Could you check a few things on this model? Use its own coordinates, in mm. Give positions to 0.01 mm unless a question says otherwise; leave off trailing zeros. Order: outer loops, then holes, each group sorted by start corner. A loop starts at its lowest first (then second) coordinate and runs counter-clockwise, first axis right, second up. Notation, with made-up numbers: (58.25, -31) -> (62.25, -31) arc R18 ccw to (62.25, -12) -> close; hole circle Ø11 at (53, -33). An arc over 180 degrees is marked (long way). Answer as CSV lines item,"result". Start each with the question number.
(1) I want a section at A-A (x = 0). Please give me the cut outline in (y, z).
(2) I want a section at B-B (z = 8.5). Please give me the cut outline in (x, y), plus the area to 3 significant figures.
(3) I need wall thicknesses on L1, parallel to Z at x = 0, y = -2.25; L2, parallel to X at y = -6, z = 9; L3, parallel to Z at x = -1.5, y = -4.5. Which ranges of each line are inside material? Lowest first, please.
(4) We'd pull the mould along Z, two halves only. Please class faces 1 (the face through (-1, -3, 38.1)), 2 (the face through (-38.1, -3, 0)), 3 (the face through (-28.204, -3.219, 0.07)): released by +Z, released by -Z, zero draft, split by the parting line, or undercut.
(5) I want a section at C-C (y = -4.25). Please give me the cut outline in (x, z) (1 decimal).
```python
from build123d import *

# Parameters (mm, degrees)
F0_W     = 76.170526
F0_H     = 75.706247
F0_R     = 14.2748
F1_DEPTH = 6.35
F2_R     = 1.5875
F3_DEPTH = 6.35
F4_R     = 1.5875
F5_DEPTH = 6.35


with BuildPart() as f1:
    # F0 (on Front) → F1 (new body)
    with BuildSketch(Plane.XZ):
        with Locations((-0.014737, 0.246877)):
            Rectangle(F0_W, F0_H)
        Circle(F0_R, mode=Mode.SUBTRACT)
    extrude(amount=F1_DEPTH)

    # F2 (on face) → F3 (cut)
    with BuildSketch(Plane.XZ.offset(6.35)):
        with Locations((-26.618414, 0)):
            Circle(F2_R)
    extrude(amount=-F3_DEPTH, mode=Mode.SUBTRACT)

    # F4 (on face) → F5 (cut)
    with BuildSketch(Plane.XZ.offset(6.35)):
        with Locations((25.999378, 0.246877)):
            Circle(F4_R)
    extrude(amount=-F5_DEPTH, mode=Mode.SUBTRACT)


solid = f1.part
```
Final values:
1,outline,"(-6.35, -37.61) -> (0, -37.61) -> (0, -14.27) -> (-6.35, -14.27) -> close; (-6.35, 14.27) -> (0, 14.27) -> (0, 38.1) -> (-6.35, 38.1) -> close"
2,outline,"(-38.1, -6.35) -> (-11.47, -6.35) -> (-11.47, 0) -> (-38.1, 0) -> close; (11.47, -6.35) -> (38.07, -6.35) -> (38.07, 0) -> (11.47, 0) -> close"
2,area,"338 mm²"
3,L1,"-37.61 to -14.27, 14.27 to 38.1"
3,L2,"-38.1 to -11.08, 11.08 to 38.07"
3,L3,"-37.61 to -14.2, 14.2 to 38.1"
4,face 1,"released by +Z"
4,face 2,"zero draft"
4,face 3,"undercut"
5,outline,"(-38.1, -37.6) -> (38.1, -37.6) -> (38.1, 38.1) -> (-38.1, 38.1) -> close; hole circle Ø3.2 at (-26.6, 0); hole circle Ø28.5 at (0, 0); hole circle Ø3.2 at (26, 0.2)"
